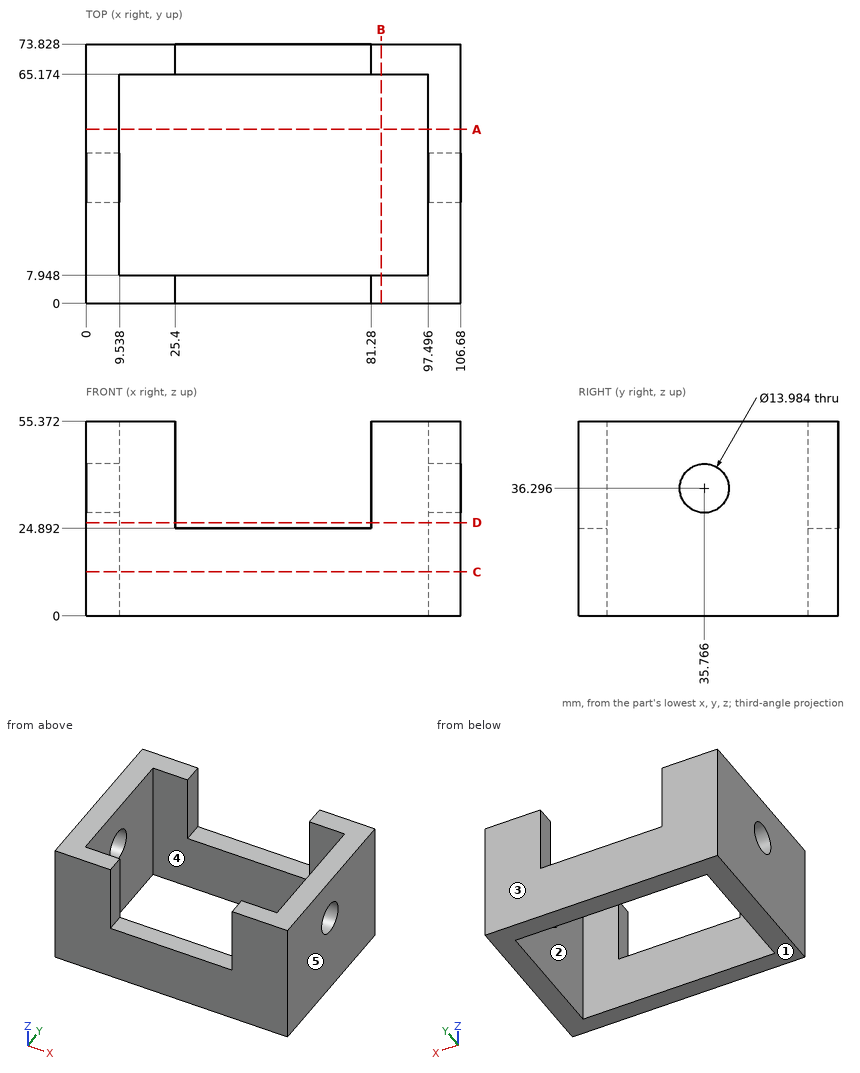
For this review, use the dimensioned drawing (mm, ordinates from the lowest corner) and the shaded views. A direction names the side the tool comes from. Coordinates: 2 decimals unless noted, no trailing zeros. Write each loop counter-clockwise with the first axis right and the second up, starting at its lowest first coordinate (ties: lowest second). Pieces come first, ordered by that corner, then holes. Notation, with made-up numbers: (81.25, 22.5) - (117.25, 22.5) arc R10 ccw to (117.25, 37.5) - close; hole circle Ø2 at (-4, 44). An arc over 180 degrees is marked (long way). One line per item, written item: value.
1) Add section A-A (y = 49.5). State the section outline as (x, z) points (1 decimal).
Answer sheet:
outline: (0, 0) - (9.5, 0) - (9.5, 55.4) - (0, 55.4) - close; (97.5, 0) - (106.7, 0) - (106.7, 55.4) - (97.5, 55.4) - close
2) Mouldability with a two-part tool opening along Y and no side actions: class the marked faces 1, 2 and 3 as +Y half, -Y half, draft (parallel to the pull), parting line (faces both ways), or undercut.
Answer sheet:
face 1: draft
face 2: undercut
face 3: +Y half
3) To check wall thickness, follow probe 1 along X at (y, z) = (6.5, 32.5); probe 2 along X at (y, z) = (30, 26) (1 decimal); probe 3 along Y at (x, z) = (53, 8). State the ranges of each line that lie inside material, in increasing order.
Answer sheet:
probe 1: x = 0 to 25.4, 81.28 to 106.68
probe 2: x = 0 to 9.5, 97.5 to 106.7
probe 3: y = 0 to 7.95, 65.17 to 73.83
4) For the marked faces 4 and 5, list the 3-axis set-ups (+Z, -Z, +X, -X, +Y, -Y) from which the entire face can be reached by the end or side of a thin tool; tool diameter is ignored.
Answer sheet:
face 4: +Z, -Z
face 5: +Z, -Z, +X, +Y, -Y
5) Add section D-D (z = 26.5). State the section outline as (x, y) points (1 decimal).
Answer sheet:
outline: (0, 0) - (25.4, 0) - (25.4, 7.9) - (9.5, 7.9) - (9.5, 65.2) - (25.4, 65.2) - (25.4, 73.8) - (0, 73.8) - close; (81.3, 0) - (106.7, 0) - (106.7, 73.8) - (81.3, 73.8) - (81.3, 65.2) - (97.5, 65.2) - (97.5, 7.9) - (81.3, 7.9) - close
6) Add section C-C (z = 12.5). State the section outline as (x, y) points (1 decimal).
Answer sheet:
outline: (0, 0) - (106.7, 0) - (106.7, 73.8) - (0, 73.8) - close; hole (9.5, 7.9) - (97.5, 7.9) - (97.5, 65.2) - (9.5, 65.2) - close
7) Insertion check: pin 1 (2.5 mm diameter, centred on x = 52.5, y = 67.5, fed in from +Z); pin 2 (8 mm diameter, centred on x = 88, y = 14.5, fed in from +Z). Each pin has a flat end and moves straight along its axis. Give the tip position at first contact, or say it passes through.
Answer sheet:
pin 1: stops at z = 24.89
pin 2: passes through
8) Add section B-B (x = 84). State the section outline as (y, z) points.
Answer sheet:
outline: (0, 0) - (7.95, 0) - (7.95, 55.37) - (0, 55.37) - close; (65.17, 0) - (73.83, 0) - (73.83, 55.37) - (65.17, 55.37) - close
